from build123d import *

# Parameters (mm, degrees)
F0_R     = 6.5
F0_R_2   = 3.5
F4_DEPTH = 1.2
F0_R_3   = 2.5
F5_DEPTH = 2.1
F6_DEPTH = 4.5
F7_R     = 0.6


# Not quite as in the source:
# - a feature names something its author has since deleted; it is built from what else it names


with BuildPart() as f4:
    # F0 (on Top) → F4 (new body)
    with BuildSketch(Plane.XY):
        Circle(F0_R)
        Circle(F0_R_2, mode=Mode.SUBTRACT)
    extrude(amount=F4_DEPTH)

    # F0 (on Top) → F5 (join)
    with BuildSketch(Plane.XY):
        Circle(F0_R_2)
        Circle(F0_R_3, mode=Mode.SUBTRACT)
    extrude(amount=F5_DEPTH)

    # F0 (on Top) → F6 (join)
    with BuildSketch(Plane.XY):
        Circle(F0_R_3)
    extrude(amount=F6_DEPTH)

    # F7
    f7_edges = [f4.edges().sort_by_distance(p)[0] for p in [
        (-2.5, 0, 4.5),
        (-6.5, 0, 0),
    ]]
    fillet(f7_edges, radius=F7_R)


solid = f4.part
For this review, take the finished solid that the model builds, in its own axes (mm). A direction names the side the tool comes from. Round coordinates to 2 decimals unless told otherwise and drop trailing zeros. Order: outer loops, then holes, each group sorted by start corner. A loop starts at its lowest first (then second) coordinate and runs counter-clockwise, first axis right, second up. Notation, with made-up numbers: (-11.5, -28.5) -> (14.5, -28.5) arc R34 ccw to (14.5, 8.5) -> close; hole circle Ø4 at (67, -14). An arc over 180 degrees is marked (long way). Write item = value, one per line. Start each with the question number.
1) To check wall thickness, follow line 1 (Z direction, x = 3.25, y = -2.5); line 2 (Z direction, x = -2.5, y = 0.5); line 3 (Y direction, x = 2.25, z = 3.8). State the ranges of each line that lie inside material, in increasing order. Write a range as from..to.
2) Take a section at C-C on z = 2.95. State the section outline as (x, y) points.
3) Take a section at A-A on y = 0. State the section outline as (x, z) points, plus the area to 3 significant figures.
4) Tool access review of faces 1 (the face through (0, 0, 4.5)), 2 (the face through (3, -3, 1.2)): name each direction out of +Z, -Z, +X, -X, +Y, -Y from which nothing blocks a thin tool from reaching the whole face with its end or side.
5) Insertion check: pin 1 (4 mm diameter, centred on x = 2, y = -3.5, fed in from +Z). The pin has a flat end and moves straight along its axis. Give the tip position at first contact, or say it passes through.
Verdict:
q1.line_1 = 0..1.2
q1.line_2 = 0..2.1
q1.line_3 = -1.09..1.09
q2.outline = circle Ø5 at (0, 0)
q3.outline = (-6.5, 0.6) arc R0.6 ccw to (-5.9, 0) -> (5.9, 0) arc R0.6 ccw to (6.5, 0.6) -> (6.5, 1.2) -> (3.5, 1.2) -> (3.5, 2.1) -> (2.5, 2.1) -> (2.5, 3.9) arc R0.6 ccw to (1.9, 4.5) -> (-1.9, 4.5) arc R0.6 ccw to (-2.5, 3.9) -> (-2.5, 2.1) -> (-3.5, 2.1) -> (-3.5, 1.2) -> (-6.5, 1.2) -> close
q3.area = 33.6 mm2
q4.face_1 = +Z, +X, -X, +Y, -Y
q4.face_2 = +Z
q5.pin_1 = 4.49
